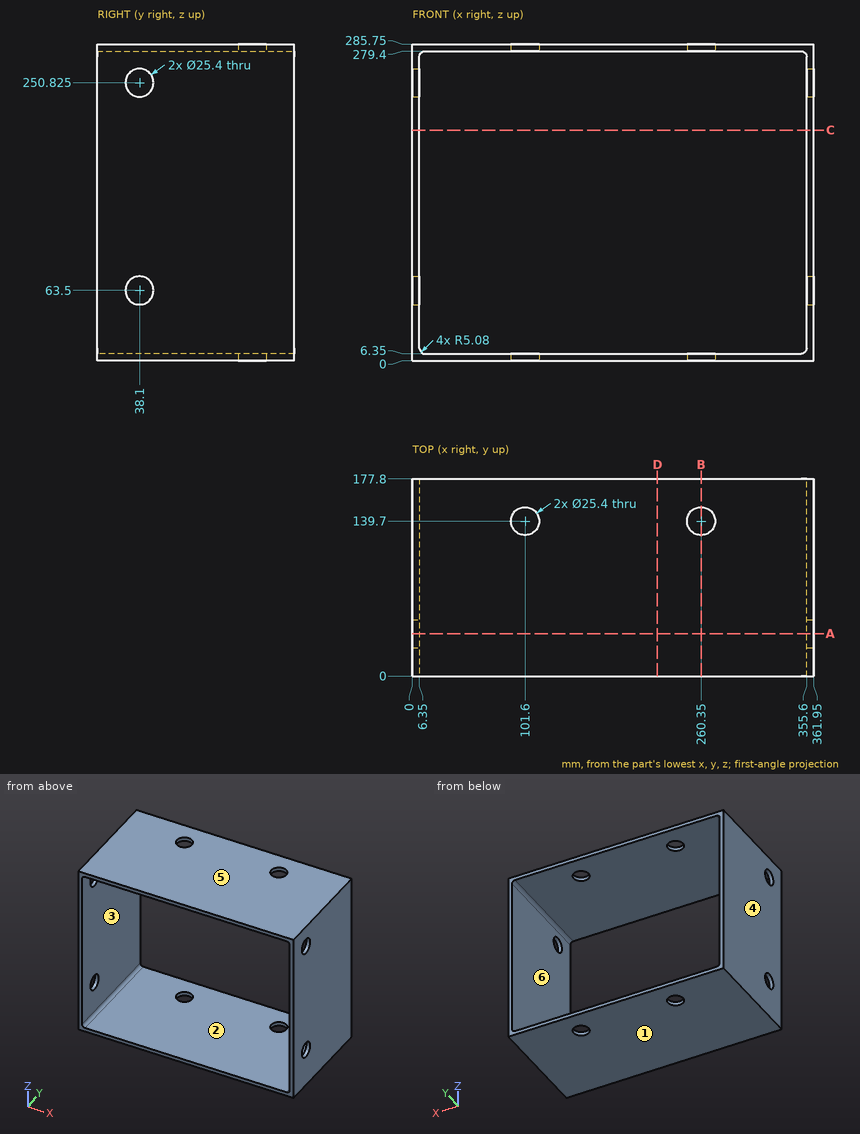
Answer from the drawing. Dimensions are ordinates in mm from the lowest x, y and z of the part. A direction names the side the tool comes from. Coordinates: 2 decimals unless noted, no trailing zeros. Write each loop counter-clockwise with the first axis right and the second up, starting at its lowest first coordinate (ties: lowest second). Pieces come first, ordered by that corner, then holes. Notation, with made-up numbers: M 71.25,-36.75 L 84.25,-36.75 A20 cw 84.25,-21.75 Z; hole C 54.5,15 d11. An arc over 180 degrees is marked long. Use a Markdown table: item, result.
Q1. This flat-tipped pin is pushed along its axis until it touches: pin 1 Ø15 at (y, z) = (38.1, 250.825) entering from -X. Where does it stop, or does it pass through?
Answer block:
| item | result |
|---|---|
| pin 1 | passes through |
Q2. Which of the six approach directions +Z, -Z, +X, -X, +Y, -Y give full straight-line access (tool end or side, diameter ignored) to the marked faces 1 and 2?
Answer block:
| item | result |
|---|---|
| face 1 | -Z, +X, -X, +Y, -Y |
| face 2 | +Y, -Y |
Q3. The part is cut by section A-A, the plane y = 38.1. Write down the section's boundary in (x, z) (3 decimals).
Answer block:
| item | result |
|---|---|
| outline | M 0,0 L 361.95,0 L 361.95,50.8 L 355.6,50.8 L 355.6,11.43 A5.08 cw 350.52,6.35 L 11.43,6.35 A5.08 cw 6.35,11.43 L 6.35,50.8 L 0,50.8 Z; M 0,76.2 L 6.35,76.2 L 6.35,238.125 L 0,238.125 Z; M 0,263.525 L 6.35,263.525 L 6.35,274.32 A5.08 cw 11.43,279.4 L 350.52,279.4 A5.08 cw 355.6,274.32 L 355.6,263.525 L 361.95,263.525 L 361.95,285.75 L 0,285.75 Z; M 355.6,76.2 L 361.95,76.2 L 361.95,238.125 L 355.6,238.125 Z |
Q4. The part is cut by section D-D, the plane x = 221. Write down the section's boundary in (y, z).
Answer block:
| item | result |
|---|---|
| outline | M 0,0 L 177.8,0 L 177.8,6.35 L 0,6.35 Z; M 0,279.4 L 177.8,279.4 L 177.8,285.75 L 0,285.75 Z |
Q5. Straight lines are drawn through the part: L1, parallel to Z at x = 360.25, y = 38.1 (3 decimals); L2, parallel to Z at x = 174.5, y = 136.5; L3, parallel to X at y = 14.5, z = 48. For each, find the intervals that lie inside material, in ascending order. Write a range as [from, to].
Answer block:
| item | result |
|---|---|
| L1 | z = [0, 50.8], [76.2, 238.125], [263.525, 285.75] |
| L2 | z = [0, 6.35], [279.4, 285.75] |
| L3 | x = [0, 6.35], [355.6, 361.95] |
Q6. The part is cut by section C-C, the plane z = 208. Write down the section's boundary in (x, y), then the cut area to 3 significant figures.
Answer block:
| item | result |
|---|---|
| outline | M 0,0 L 6.35,0 L 6.35,177.8 L 0,177.8 Z; M 355.6,0 L 361.95,0 L 361.95,177.8 L 355.6,177.8 Z |
| area | 2,260 mm2 |
Q7. Determine the mould class of the marked faces 3, 4, 5 and 6 for opening direction Z: released by +Z, released by -Z, zero draft, split by the parting line, or undercut.
Answer block:
| item | result |
|---|---|
| face 3 | undercut |
| face 4 | zero draft |
| face 5 | released by +Z |
| face 6 | undercut |
Q8. The part is cut by section B-B, the plane x = 260.35. Write down the section's boundary in (y, z), then the cut area to 3 significant figures.
Answer block:
| item | result |
|---|---|
| outline | M 0,0 L 127,0 L 127,6.35 L 0,6.35 Z; M 0,279.4 L 127,279.4 L 127,285.75 L 0,285.75 Z; M 152.4,0 L 177.8,0 L 177.8,6.35 L 152.4,6.35 Z; M 152.4,279.4 L 177.8,279.4 L 177.8,285.75 L 152.4,285.75 Z |
| area | 1,940 mm2 |
